Can you work these out from the model? Positions are in its coordinate system, mm. Face numbers are marked on the shaded views. A direction names the side the tool comes from. Coordinates: 2 decimals unless noted, no trailing zeros. Order: outer loops, then holes, each group sorted by start corner. A loop starts at its lowest first (then second) coordinate and runs counter-clockwise, first axis right, second up.
Autodesk Fusion 360 part; units mm, degrees
sketch "Szkic1" plane through (0, 0, 0) normal (0, 0, 1) x (1, 0, 0)
  line L0 (0, 0) -> (12.4, 0)
  line L1 (12.4, 0) -> (12.4, 22.6)
  line L2 (12.4, 22.6) -> (0, 22.6)
  line L3 (0, 22.6) -> (0, 0)
  dimension "d1" = 12.4
  dimension "d2" = 22.6
extrude "Wyciągnięcie proste1" add sketch "Szkic1" along normal blind 15.8
sketch "Szkic2" plane through (0, 0, 15.8) normal (0, 0, 1) x (-1, 0, 0)
  line L0 (0, -22.6) -> (0, 0)
  line L1 (0, 0) -> (-12.4, 0)
  line L2 (-12.4, 0) -> (-12.4, -22.6)
  line L3 (-12.4, -22.6) -> (0, -22.6)
  line L4 (0, 0) -> (0, 4.85)
  line L5 (0, 0) -> (0, -11.3)
  line L6 (0, -11.3) -> (-12.4, -11.3)
  line L7 (0, 4.85) -> (-12.4, 4.85)
  line L8 (-12.4, 4.85) -> (-12.4, 0)
  line L9 (0, 0) -> (-6.2, 0)
  line L10 (-6.2, 0) -> (-6.2, 2.7)
  circle A0 centre (-6.2, 2.7) radius 1.1
  line L11 (-6.2, 2.7) -> (-6.2, 4.85)
  line L12 (-6.2, 4.85) -> (-6.85, 4.85)
  line L13 (-6.85, 4.85) -> (-6.85, 3.5874)
  line L14 (-5.55, 4.85) -> (-5.55, 3.5874)
  line L15 (-6.2, -27.45) -> (-6.85, -27.45)
  line L16 (-6.2, -22.6) -> (-6.2, -25.3)
  line L17 (0, -22.6) -> (0, -27.45)
  line L18 (-12.4, -27.45) -> (-12.4, -22.6)
  line L19 (-6.2, -25.3) -> (-6.2, -27.45)
  line L20 (-6.85, -27.45) -> (-6.85, -26.1874)
  line L21 (0, -27.45) -> (-12.4, -27.45)
  line L22 (-5.55, -27.45) -> (-5.55, -26.1874)
  line L23 (0, -22.6) -> (-6.2, -22.6)
  line L24 (0, 0) -> (0, -22.6)
  circle A1 centre (-6.2, -25.3) radius 1.1
  line L25 (0, -22.6) -> (-12.4, -22.6)
  line L26 (-12.4, -22.6) -> (-12.4, 0)
  line L27 (0, -22.6) -> (0, -11.3)
  point P0 (0, -22.6)
  dimension "d5" = 4.85
  dimension "d6" = 2.7
  dimension "d7" = 2.2
  dimension "d8" = 0.65
extrude "Wyciągnięcie proste2" add sketch "Szkic2" along normal blind 2.2 contours L0 L2 L3 L6 L23 L24 L25 L26 L27 | L3 L16 L17 L21 L22 L23 A1 L25 | L0 L1 L2 L5 L6 L9 L24 L26 | L3 L16 L18 L20 L21 A1 L25 | L1 L4 L7 L9 L10 A0 L14 | L1 L7 L8 L10 A0 L13
extrude "Wyciągnięcie proste3" add sketch "Szkic1" along normal blind 22
sketch "Szkic3" plane through (0, 0, 22) normal (0, 0, 1) x (-1, 0, 0)
  line L0 (0, -22.6) -> (0, 0)
  line L1 (0, 0) -> (-12.4, 0)
  line L2 (-12.4, 0) -> (-12.4, -22.6)
  line L3 (-12.4, -22.6) -> (0, -22.6)
  line L4 (-12.4, 0) -> (-12.4, -12.4)
  line L5 (-12.4, -12.4) -> (-12.4, -12)
  line L6 (0, 0) -> (-1, -1)
  line L7 (-12.4, 0) -> (-12.4, -11.3)
  line L8 (-12.4, -12.4) -> (-8.85, -12.4)
  line L9 (-3.55, -12.4) -> (0, -12.4)
  arc A0 (-3.6112, -11.8337) -> (-8.7888, -11.8337) centre (-6.2, -6.2) ccw
  arc A1 (-8.7888, -11.8337) -> (-3.6112, -11.8337) centre (-6.2, -12.4) ccw
  line L10 (-1, -1) -> (-1.8159, -1.8159)
  line L11 (-10.5841, -10.5841) -> (-12.4, -12.4)
  line L12 (0, -12.4) -> (-1.8159, -10.5841)
  line L13 (-10.5841, -1.8159) -> (-12.4, 0)
  dimension "d13" = 12.4
  dimension "d14" = 11.3
  dimension "d15" = 5.3
extrude "Wyciągnięcie proste4" add sketch "Szkic3" along normal blind 4.2 contours A0 A1
sketch "Szkic4" plane through (0, 0, 26.2) normal (0, 0, 1) x (-1, 0, 0)
  arc A0 (-8.7888, -11.8337) -> (-3.6112, -11.8337) centre (-6.2, -12.4) ccw
  arc A1 (-3.6112, -11.8337) -> (-8.7888, -11.8337) centre (-6.2, -6.2) ccw
  circle A2 centre (-6.2, -6.2) radius 3.35
  dimension "d18" = 6.7
extrude "Wyciągnięcie proste5" add sketch "Szkic4" along normal blind 3 contours A2
sketch "Szkic5" plane through (0, 0, 29.2) normal (0, 0, 1) x (-1, 0, 0)
  circle A0 centre (-6.2, -6.2) radius 3.35
  line L0 (-6.2, -6.2) -> (-6.2, -22.2)
  line L1 (-6.2, -6.2) -> (-6.2, 9.8)
  line L2 (-6.2, -22.2) -> (-6.2, -20.2)
  circle A1 centre (-6.2, -20.2) radius 0.5
  circle A2 centre (-6.2, -18.2) radius 0.5
  circle A3 centre (-6.2, -16.2) radius 0.5
  circle A4 centre (-6.2, -14.2) radius 0.5
  circle A5 centre (-6.2, -12.2) radius 0.5
  circle A6 centre (-6.2, -10.2) radius 0.5
  line L3 (-6.2, -6.2) -> (-9, -6.2)
  circle A7 centre (-6.2, 1.8) radius 0.5
  circle A8 centre (-6.2, -0.2) radius 0.5
  circle A9 centre (-6.2, 5.8) radius 0.5
  circle A10 centre (-6.2, 3.8) radius 0.5
  circle A11 centre (-6.2, -2.2) radius 0.5
  circle A12 centre (-6.2, 7.8) radius 0.5
  circle A13 centre (-6.2, -6.2) radius 3.35
  line L4 (-6.2, -6.2) -> (-6.2, -6.5)
  line L5 (-6.2, -9.55) -> (-8.9, -9.55)
  line L6 (-6.2, -20.2) -> (-8.2, -20.2)
  line L7 (-8.9, -9.55) -> (-8.2, -20.2)
  line L8 (-8.9, -9.55) -> (-8.9348, -9.0209)
  line L9 (-8.9348, -9.0209) -> (-8.9992, -8.0403)
  line L10 (-6.2, -9.55) -> (-3.5, -9.55)
  line L11 (-3.5, -9.55) -> (-4.2, -20.2)
  circle A14 centre (-6.2, -6.2) radius 3.35
  circle A15 centre (-6.2, -6.2) radius 3.35
  line L12 (-3.5, -9.55) -> (-3.4652, -9.0209)
  line L13 (-6.2, -20.2) -> (-4.2, -20.2)
  line L14 (-3.4652, -9.0209) -> (-3.4008, -8.0403)
  arc A16 (-8.2, -20.2) -> (-4.2, -20.2) centre (-6.2, -20.2) ccw
  line L15 (-6.2, 9.8) -> (-6.2, 7.8)
  line L16 (-6.2, -2.85) -> (-8.9, -2.85)
  circle A17 centre (-6.2, 3.8) radius 0.5
  line L17 (-3.5, -2.85) -> (-4.2, 7.8)
  circle A18 centre (-6.2, 1.8) radius 0.5
  line L18 (-6.2, 7.8) -> (-8.2, 7.8)
  circle A19 centre (-6.2, 5.8) radius 0.5
  line L19 (-8.9, -2.85) -> (-8.2, 7.8)
  line L20 (-8.9, -2.85) -> (-8.9348, -3.3791)
  arc A20 (-4.2, 7.8) -> (-8.2, 7.8) centre (-6.2, 7.8) ccw
  line L21 (-6.2, 7.8) -> (-4.2, 7.8)
  circle A21 centre (-6.2, 7.8) radius 0.5
  line L22 (-3.5, -2.85) -> (-3.4652, -3.3791)
  line L23 (-3.4652, -3.3791) -> (-3.4008, -4.3597)
  line L24 (-8.9348, -3.3791) -> (-8.9992, -4.3597)
  line L25 (-6.2, -2.85) -> (-3.5, -2.85)
  circle A22 centre (-6.2, -0.2) radius 0.5
  circle A23 centre (-6.2, -2.2) radius 0.5
  point P0 (-6.2, 7.8)
  dimension "d21" = 16
  dimension "d22" = 16
  dimension "d23" = 2
  dimension "d24" = 1
  dimension "d27" = 0
  dimension "d28" = 10
  dimension "d29" = 6.7
  dimension "d30" = 2.7
  dimension "d31" = 2
extrude "Wyciągnięcie proste6" add sketch "Szkic5" along normal blind 1.5 contours A0 L0 L1 A13 L4 A14 A15 | A0 A13 A14 A15 L22 L23 L25 | A0 A13 L10 A14 A15 L12 L14 | A0 L0 L1 A13 L4 A14 A15 | L1 A7 A8 A9 A10 A11 A12 L16 A17 A18 L18 A19 L19 A21 A22 A23 | A0 A13 A14 A15 L16 L20 L24 | L1 A7 A8 A9 A10 A11 A12 A17 L17 A18 A19 L21 A21 L25 A22 A23 | A0 A13 L5 L8 L9 A14 A15 | L0 A1 A2 A3 A4 A5 A6 L10 L11 L13 | L0 A1 A2 A3 A4 A5 A6 L5 L6 L7 | L1 A12 L15 L18 A20 A21 | L1 A12 L15 A20 L21 A21 | L0 L2 A1 L6 A16 | L0 L2 A1 L13 A16
equation "d5 = ( ( 32.3 - 22.6 ) / 2 ) * 1 mm"
equation "d6 = ( ( 28 - 22.6 ) / 2 ) * 1 mm"
equation "d8 = ( 1.3 / 2 ) * 1 mm"
equation "d30 = ( 5.4 / 2 ) * 1 mm"
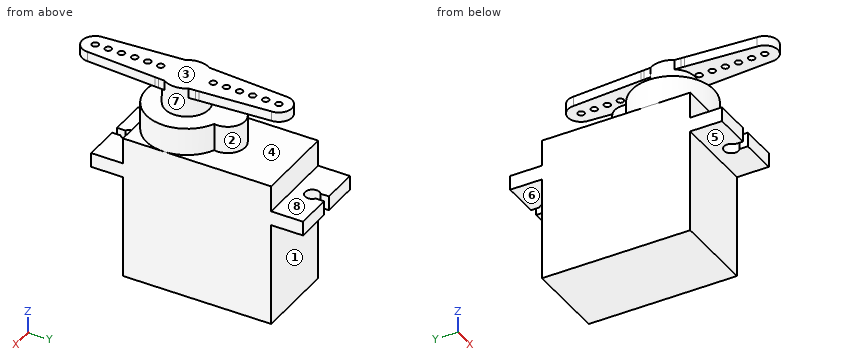
1. Imagine slicing it at C-C on y = 14.2. Please give me the cut outline in (x, z).
Completed:
outline: (0, 0) - (12.4, 0) - (12.4, 22) - (8.14, 22) - (8.14, 26.2) - (4.26, 26.2) - (4.26, 22) - (0, 22) - close; (3.81, 29.2) - (5.7, 29.2) - (5.7, 30.7) - (3.81, 30.7) - close; (6.7, 29.2) - (8.59, 29.2) - (8.59, 30.7) - (6.7, 30.7) - close
2. On a 3-axis mill with a long thin cutter (end or side, diameter ignored), from which of +Z, -Z, +X, -X, +Y, -Y can I reach the whole of each face in a straight line? I mean the marked faces 4, 5, 6, 7 and 8. Say none if no direction works.
Completed:
face 4: +Y
face 5: -Z, +X, -X, -Y
face 6: -Z, +X, -X, +Y
face 7: none
face 8: +Z, +X, -X, +Y
3. Imagine slicing it at B-B on z = 17. Please give me the cut outline in (x, y).
Completed:
outline: (0, -4.85) - (5.55, -4.85) - (5.55, -3.59) arc R1.1 cw (long way) to (6.85, -3.59) - (6.85, -4.85) - (12.4, -4.85) - (12.4, 27.45) - (6.85, 27.45) - (6.85, 26.19) arc R1.1 cw (long way) to (5.55, 26.19) - (5.55, 27.45) - (0, 27.45) - close
4. Thinking about a two-plate mould opening in Z: for the marked faces 1, 2 and 3, which applies, pulls with the +Z half, pulls with the -Z half, needs draft (parallel to the pull), parting line crosses it, or undercut?
Completed:
face 1: needs draft
face 2: undercut
face 3: pulls with the +Z half
5. Please list where these lines run through material, in increasing order: probe 1 along Z at (x, y) = (5.5, 17); probe 2 along Z at (x, y) = (4, 1); probe 3 along X at (y, z) = (-2.7, 16.4).
Completed:
probe 1: z = 0 to 22, 29.2 to 30.7
probe 2: z = 0 to 26.2, 29.2 to 30.7
probe 3: x = 0 to 5.1, 7.3 to 12.4
6. Imagine slicing it at D-D on x = 1.75. Please give me the cut outline in (y, z), then the cut area to 3 significant figures.
Completed:
outline: (-4.85, 15.8) - (0, 15.8) - (0, 0) - (22.6, 0) - (22.6, 15.8) - (27.45, 15.8) - (27.45, 18) - (22.6, 18) - (22.6, 22) - (10.52, 22) - (10.52, 26.2) - (1.88, 26.2) - (1.88, 22) - (0, 22) - (0, 18) - (-4.85, 18) - close
area: 555 mm2
7. I'm going to push flat-ended pins straight in: pin 1 (2 mm diameter, centred on x = 11, z = 8, fed in from +Y); pin 2 (2.5 mm diameter, centred on x = 6.2, y = -2.7, fed in from -Z); pin 3 (1 mm diameter, centred on x = 7.5, z = 25, fed in from -Y). Where does each tip first touch, or does it pass through?
Completed:
pin 1: stops at y = 22.6
pin 2: stops at z = 15.8
pin 3: stops at y = 0.05
8. Imagine slicing it at A-A on y = 25.3. Please give me the cut outline in (x, z).
Completed:
outline: (0, 15.8) - (5.1, 15.8) - (5.1, 18) - (0, 18) - close; (7.3, 15.8) - (12.4, 15.8) - (12.4, 18) - (7.3, 18) - close
